Check sheet for the drawn part. Datum: minimum x, y, z corner. Units: mm. A direction names the side the tool comes from. Give positions to 0.01 mm unless a question says otherwise; leave off trailing zeros. Loops run counter-clockwise (first coordinate to the right, second up) from the corner with the lowest first, then second, coordinate; pieces in that order, holes last. Notation, with made-up numbers: (-27, 31) - (-12, 31) arc R14 cw to (-12, 45) - close; hole circle Ø1 at (74.25, 69). An arc over 180 degrees is marked (long way). Use a Markdown table: item, result. Add a question column.
1. Cross-section at C-C on z = 0.95. Enter the section's corners in (x, y), and give its area (3 significant figures).
2. Depth check by flat-ended pin: P1, Ø4, axis at x = 10.5, y = 5, coming from the +Z side. Enter the tip coordinate at first touch or a pass-through.
3. Cross-section at B-B on x = 8.25. Enter the section's corners in (y, z).
4. Material ranges on L1, parallel to Y at x = 8.25, z = 2.15; L2, parallel to X at y = 4, z = 0.95; L3, parallel to Y at x = 13, z = 2.3, recorded low to high.
5. Cross-section at A-A on y = 5. Enter the section's corners in (x, z), and give its area (3 significant figures).
6. Set-up check for the marked faces 5 and 6: record each of +Z, -Z, +X, -X, +Y, -Y from which the full face is reachable in a straight line by a thin tool's end or side.
7. Cross-section at D-D on y = 14. Enter the section's corners in (x, z), and give its area (4 significant figures).
8. Draft check along Y on the marked faces 1, 2, 3 and 4. Enter one of: pulls with the +Y half, pulls with the -Y half, needs draft (parallel to the pull), parting line crosses it, or undercut.
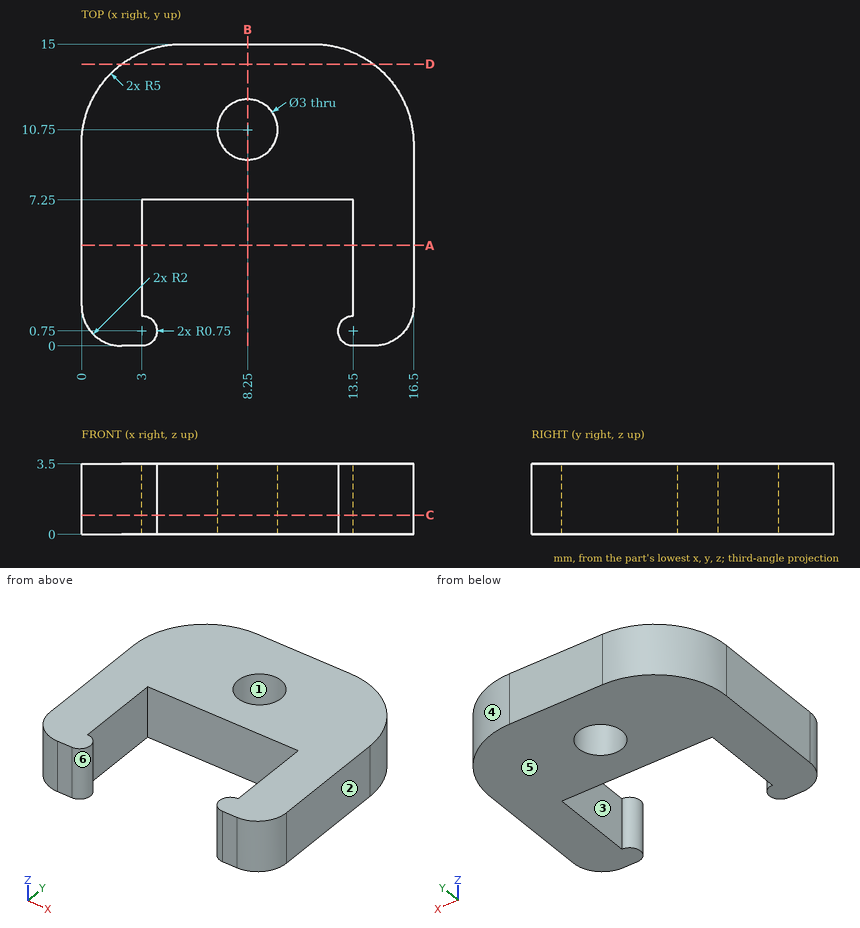
Values found:
| question | item | result |
|---|---|---|
| 1 | outline | (0, 2) arc R2 ccw to (2, 0) - (3, 0) arc R0.75 ccw to (3, 1.5) - (3, 7.25) - (13.5, 7.25) - (13.5, 1.5) arc R0.75 ccw to (13.5, 0) - (14.5, 0) arc R2 ccw to (16.5, 2) - (16.5, 10) arc R5 ccw to (11.5, 15) - (5, 15) arc R5 ccw to (0, 10) - close; hole circle Ø3 at (8.25, 10.75) |
| 1 | area | 154 mm2 |
| 2 | P1 | passes through |
| 3 | outline | (7.25, 0) - (9.25, 0) - (9.25, 3.5) - (7.25, 3.5) - close; (12.25, 0) - (15, 0) - (15, 3.5) - (12.25, 3.5) - close |
| 4 | L1 | y = 7.25 to 9.25, 12.25 to 15 |
| 4 | L2 | x = 0 to 3, 13.5 to 16.5 |
| 4 | L3 | y = 0.19 to 1.31, 7.25 to 14.77 |
| 5 | outline | (0, 0) - (3, 0) - (3, 3.5) - (0, 3.5) - close; (13.5, 0) - (16.5, 0) - (16.5, 3.5) - (13.5, 3.5) - close |
| 5 | area | 21.0 mm2 |
| 6 | face 5 | -Z, +X, -X, +Y, -Y |
| 6 | face 6 | +Z, -Z |
| 7 | outline | (2, 0) - (14.5, 0) - (14.5, 3.5) - (2, 3.5) - close |
| 7 | area | 43.75 mm2 |
| 8 | face 1 | undercut |
| 8 | face 2 | needs draft |
| 8 | face 3 | undercut |
| 8 | face 4 | pulls with the +Y half |
